Build history of the part. All positions in model axes, mm. A direction names the side the tool comes from. Round coordinates to 2 decimals unless told otherwise and drop trailing zeros. Write each loop counter-clockwise with the first axis right and the second up, starting at its lowest first coordinate (ties: lowest second). Pieces come first, ordered by that corner, then holes. Notation, with made-up numbers: (-5, 13) - (5, 13) arc R21 cw to (5, 34) - close; hole circle Ø5 at (-10, -31.75). An arc over 180 degrees is marked (long way). Write each question's results on one line, items separated by ' | '.
from build123d import *

# Parameters (mm, degrees)
SOFT_CONTACT_AND_WRAP_START      = -1
SOFT_CONTACT_AND_WRAP_PROFILE_W  = 14
SOFT_CONTACT_AND_WRAP_PROFILE_H  = 7
SOFT_CONTACT_AND_WRAP_DEPTH      = 7
FINGER_SLIP_POCKET_PROFILE_W     = 12.2
FINGER_SLIP_POCKET_PROFILE_H     = 5.2
OPEN_TOP_SLIP_POCKET_DEPTH       = 7
SERVO_EAR_SWEEP_RELIEF_START     = 3.8
SERVO_EAR_SWEEP_RELIEF_PROFILE_W = 16
SERVO_EAR_SWEEP_RELIEF_PROFILE_H = 3
SERVO_EAR_SWEEP_RELIEF_DEPTH     = 3.2
PAD_CAPTURE_M2_START             = -50
PAD_CAPTURE_M2_PROFILE_R         = 1.1
PAD_CAPTURE_M2_DEPTH             = 86.510561809


with BuildPart() as part:
    # Soft_contact_and_wrap_profile → Soft_contact_and_wrap (new body)
    with BuildSketch(Plane.XY.offset(SOFT_CONTACT_AND_WRAP_START)):
        with Locations((21, -17.5)):
            Rectangle(SOFT_CONTACT_AND_WRAP_PROFILE_W, SOFT_CONTACT_AND_WRAP_PROFILE_H)
    extrude(amount=SOFT_CONTACT_AND_WRAP_DEPTH)

    # Finger_slip_pocket_profile → Open_top_slip_pocket (cut)
    with BuildSketch(Plane.XY):
        with Locations((21, -17.5)):
            Rectangle(FINGER_SLIP_POCKET_PROFILE_W, FINGER_SLIP_POCKET_PROFILE_H)
    extrude(amount=OPEN_TOP_SLIP_POCKET_DEPTH, mode=Mode.SUBTRACT)

    # Servo_ear_sweep_relief_profile → Servo_ear_sweep_relief (cut)
    with BuildSketch(Plane.XY.offset(SERVO_EAR_SWEEP_RELIEF_START)):
        with Locations((21, -14.5)):
            Rectangle(SERVO_EAR_SWEEP_RELIEF_PROFILE_W, SERVO_EAR_SWEEP_RELIEF_PROFILE_H)
    extrude(amount=SERVO_EAR_SWEEP_RELIEF_DEPTH, mode=Mode.SUBTRACT)

    # Pad_capture_M2_profile → Pad_capture_M2 (cut, through all)
    with BuildSketch(Plane.XY.offset(PAD_CAPTURE_M2_START)):
        with Locations(Location((18, -17.5, 0), (0, 0, 180))):
            Circle(PAD_CAPTURE_M2_PROFILE_R)
        with Locations(Location((24, -17.5, 0), (0, 0, 180))):
            Circle(PAD_CAPTURE_M2_PROFILE_R)
    extrude(amount=PAD_CAPTURE_M2_DEPTH, mode=Mode.SUBTRACT)


solid = part.part
(1) Tool access for faces 4 (the flat face through (21, -14, 1)), 5 (the flat face through (21, -17, 0)), 6 (the flat face through (20.9, -14.5, 3.8)): list every direction of +Z, -Z, +X, -X, +Y, -Y with a clear straight run to the whole face (end or side of a thin tool).
Worked answers:
face 4: +Z, -Z, +X, -X, +Y | face 5: +Z | face 6: +Z, +X, -X, +Y
(2) Drill centre lines: probe 1 along Y at (x, z) = (19.5, 0.5); probe 2 along Y at (x, z) = (18, -0.3); probe 3 along X at (y, z) = (-16.5, 2.25). Where is each one in solid material? Low to high. Write a range as [from, to].
Worked answers:
probe 1: y = [-21, -20.1], [-14.9, -14] | probe 2: y = [-21, -18.6], [-16.4, -14] | probe 3: x = [14, 14.9], [27.1, 28]
(3) Slice it at B-B, the plane y = -17.5. Write the cut outline in (x, z).
Worked answers:
outline: (14, -1) - (16.9, -1) - (16.9, 0) - (14.9, 0) - (14.9, 6) - (14, 6) - close; (19.1, -1) - (22.9, -1) - (22.9, 0) - (19.1, 0) - close; (25.1, -1) - (28, -1) - (28, 6) - (27.1, 6) - (27.1, 0) - (25.1, 0) - close
(4) Slice it at A-A, the plane x = 24. Write the cut outline in (y, z), and give its area (3 significant figures).
Worked answers:
outline: (-21, -1) - (-18.6, -1) - (-18.6, 0) - (-20.1, 0) - (-20.1, 6) - (-21, 6) - close; (-16.4, -1) - (-14, -1) - (-14, 3.8) - (-14.9, 3.8) - (-14.9, 0) - (-16.4, 0) - close | area: 13.6 mm2
(5) Slice it at D-D, the plane y = -15.75. Write the cut outline in (x, z), and give its area (3 significant figures).
Worked answers:
outline: (14, -1) - (28, -1) - (28, 3.8) - (27.1, 3.8) - (27.1, 0) - (14.9, 0) - (14.9, 3.8) - (14, 3.8) - close | area: 20.8 mm2
(6) Flat gauge pins, fed straight in: pin 1 Ø0.6 at (x, y) = (19, -15) entering from +Z; pin 2 Ø0.7 at (x, z) = (27.5, 4.5) entering from +Y; pin 3 Ø2.5 at (x, y) = (22.5, -17.5) entering from +Z. Where does each tip first touch, or does it go through?
Worked answers:
pin 1: stops at z = 3.8 | pin 2: stops at y = -16 | pin 3: stops at z = 0
(7) Two-plate mould, pull along Y, no slides. Class faces 1 (the flat face through (27.5, -16, 4.9)), 2 (the flat face through (14, -18, 2)), 3 (the flat face through (27.1, -18, 3)): released by +Y, released by -Y, zero draft, split by the parting line, or undercut.
Worked answers:
face 1: released by +Y | face 2: zero draft | face 3: undercut
(8) Slice it at C-C, the plane z = 1.75. Write the cut outline in (x, y).
Worked answers:
outline: (14, -21) - (28, -21) - (28, -14) - (14, -14) - close; hole (14.9, -20.1) - (27.1, -20.1) - (27.1, -14.9) - (14.9, -14.9) - close
